from build123d import *

# Parameters (mm, degrees)
SKETCH1_W           = 44.1
SKETCH1_H           = 58.9
BOSS_EXTRUDE1_DEPTH = 1.5
CUT_EXTRUDE1_REACH  = 38.821
SKETCH2_W           = 2
SKETCH2_H           = 29.45


with BuildPart() as part:
    # Sketch1 → Boss-Extrude1 (new body)
    with BuildSketch(Plane(origin=(0, 0, 0), x_dir=(1, 0, 0), z_dir=(0, 1, 0))):
        Rectangle(SKETCH1_W, SKETCH1_H)
    extrude(amount=BOSS_EXTRUDE1_DEPTH)

    # Sketch2 → Cut-Extrude1 (cut, up to next)
    with BuildSketch(Plane(origin=(0, 1.5, 0), x_dir=(1, 0, 0), z_dir=(0, 1, 0)), mode=Mode.PRIVATE) as cut_extrude1_sk1:
        with Locations((0, 14.725)):
            Rectangle(SKETCH2_W, SKETCH2_H)
    cut_extrude1_tool1 = extrude(cut_extrude1_sk1.sketch, amount=-CUT_EXTRUDE1_REACH, mode=Mode.PRIVATE) & part.part
    add(cut_extrude1_tool1.solids().sort_by_distance((0, 1.5, -14.725))[0], mode=Mode.SUBTRACT)


solid = part.part
Here's how the part is built. I have some questions about the finished solid (model axes, mm). A direction names the side the tool comes from. Coordinates: 2 decimals unless noted, no trailing zeros. Loops run counter-clockwise (first coordinate to the right, second up) from the corner with the lowest first, then second, coordinate; pieces in that order, holes last. Notation, with made-up numbers: (72, 28.5) -> (88, 28.5) arc R22 ccw to (88, 44.5) -> close; hole circle Ø1 at (35, 24.5). An arc over 180 degrees is marked (long way). Use one line per item in the form item = value. Start each with the question number.
(1) If we section it at B-B (y = 0.35): Please give me the cut outline in (x, z).
(2) Please list where this line runs through material, in increasing order: line 1 along X through (y, z) = (0.45, -3).
(3) We'd pull the mould along X, two halves only. Please class faces 3 (the face through (5, 0, 0)), 4 (the face through (-1, 1, -15)), 5 (the face through (-22.05, 1, 0)): pulls with the +X half, pulls with the -X half, needs draft (parallel to the pull), parting line crosses it, or undercut.
(4) Will this pin go through, and if not, where does the flat tip stop? pin 1 (5 mm diameter, centred on x = 12.5, z = 0, fed in from -Y).
(5) If we section it at A-A (z = -2): Please give me the cut outline in (x, y), then the cut area to 4 significant figures.
(6) On a 3-axis mill with a long thin cutter (end or side, diameter ignored), from which of +Z, -Z, +X, -X, +Y, -Y can I reach the whole of each face in a straight line? I mean faces 1 (the face through (0, 1, 29.45)), 2 (the face through (0, 1, 0)). Say none if no direction works.
Verdict:
q1.outline = (-22.05, -29.45) -> (-1, -29.45) -> (-1, 0) -> (1, 0) -> (1, -29.45) -> (22.05, -29.45) -> (22.05, 29.45) -> (-22.05, 29.45) -> close
q2.line_1 = -22.05 to -1, 1 to 22.05
q3.face_3 = needs draft
q3.face_4 = undercut
q3.face_5 = pulls with the -X half
q4.pin_1 = 0
q5.outline = (-22.05, 0) -> (-1, 0) -> (-1, 1.5) -> (-22.05, 1.5) -> close; (1, 0) -> (22.05, 0) -> (22.05, 1.5) -> (1, 1.5) -> close
q5.area = 63.15 mm²
q6.face_1 = +Z, +X, -X, +Y, -Y
q6.face_2 = -Z, +Y, -Y
